from build123d import *

# Parameters (mm, degrees)
SKETCH1_R           = 2.921
BOSS_EXTRUDE1_DEPTH = 2.54
SKETCH3_R           = 0.762
CUT_EXTRUDE1_DEPTH  = 0.254
FILLET1_R           = 1.27
SCALE1_SCALE        = 2.43
SCALE3_SCALE        = 1.15


with BuildPart() as part:
    # Sketch1 → Boss-Extrude1 (new body)
    with BuildSketch(Plane.XY):
        with BuildLine():
            Line((0, 0), (5.08, 0))
            ThreePointArc((5.08, 0), (5.715, 6.285851973), (3.835659211, 0.254))
            Line((3.835659211, 0.254), (0, 0.254))
            Line((0, 0.254), (0, 0))
        make_face()
        with Locations((5.08, 3.175)):
            Circle(SKETCH1_R, mode=Mode.SUBTRACT)
    extrude(amount=BOSS_EXTRUDE1_DEPTH)

    # Sketch3 → Cut-Extrude1 (cut)
    with BuildSketch(Plane(origin=(0, 0.254, 0), x_dir=(1, 0, 0), z_dir=(0, 1, 0))):
        with Locations(Location((1.4605, -1.27, 0), (0, 0, 180))):
            Circle(SKETCH3_R)
    extrude(amount=-CUT_EXTRUDE1_DEPTH, mode=Mode.SUBTRACT)

    # Fillet1
    fillet1_edges = [part.edges().sort_by_distance(p)[0] for p in [
        (0, 0.127, 2.54),
        (0, 0.127, 0),
    ]]
    fillet(fillet1_edges, radius=FILLET1_R - 0.0001)  # a hair under: the kernel refuses the full size


with BuildPart() as part_1:
    # Scale1: scaled about (4.695948506, 2.731518553, 1.27)
    add(part.part.scale(SCALE1_SCALE).moved(Location((-6.715206364, -3.906071531, -1.8161))))


with BuildPart() as part_2:
    # Scale3: scaled about (4.695948505, 2.731518554, 1.27)
    add(part_1.part.scale(SCALE3_SCALE).moved(Location((-0.704392276, -0.409727783, -0.1905))))


solid = part_2.part
Could you check a few things on this model? Use its own coordinates, in mm. A direction names the side the tool comes from. Give positions to 0.01 mm unless a question says otherwise; leave off trailing zeros. Loops run counter-clockwise (first coordinate to the right, second up) from the corner with the lowest first, then second, coordinate; pieces in that order, holes last. Notation, with made-up numbers: (-10, 29.5) -> (7, 29.5) arc R21 ccw to (7, 67.5) -> close; hole circle Ø7 at (42.5, 82.5). An arc over 180 degrees is marked (long way). Return JSON: item names as keys, results as strings.
Item 1: We'd pull the mould along X, two halves only. Please class faces 4 (the cylindrical face through (-7.415, -4.552, -1.212)), 5 (the flat face through (0, -4.902, 1)), 6 (the cylindrical face through (-0.708, -0.996, 1.22)): +X half, -X half, draft (parallel to the pull), parting line (faces both ways), or undercut.
Geometry results:
{"face 4": "-X half", "face 5": "draft", "face 6": "undercut"}
Item 2: Which directions (+Z, -Z, +X, -X, +Y, -Y) give clear straight access to the entire face, cutting with the end or side of a thin tool? Please do faces 1 (the flat face through (-2, -4.192, 1)), 2 (the cylindrical face through (-6.31, -4.54, 0.45)), 3 (the flat face through (3, -4, 4.819)).
Geometry results:
{"face 1": "+Z, -Z, -X", "face 2": "-Y", "face 3": "+Z, +X, -X, +Y, -Y"}
Item 3: I'm going to push flat-ended pins straight in: pin 1 (8 mm diameter, centred on x = -4, y = 2.5, fed in from -Z); pin 2 (3 mm diameter, centred on y = 8, z = -1.5, fed in from -X); pin 3 (1 mm diameter, centred on y = 1, z = 4, fed in from +X); pin 4 (10 mm diameter, centred on x = 5.5, y = 5, fed in from +Z). Where does each tip first touch, or does it pass through?
Geometry results:
{"pin 1": "stops at z = -2.28", "pin 2": "stops at x = -2.74", "pin 3": "stops at x = 14.29", "pin 4": "passes through"}
Item 4: If we section it at C-C on x = 4.5: List the corners of the cut face in (y, z) for me.
Geometry results:
{"outline": "(-4.9, -2.28) -> (-4.09, -2.28) -> (-4.09, 4.82) -> (-4.9, 4.82) -> close; (12.03, -2.28) -> (12.75, -2.28) -> (12.75, 4.82) -> (12.03, 4.82) -> close"}
Item 5: If we section it at A-A on z = 2: List the corners of the cut face in (x, y) for me.
Geometry results:
{"outline": "(-8.35, -4.9) -> (-6.35, -4.9) -> (-6.35, -4.19) -> (-8.35, -4.19) -> close; (-2.35, -4.9) -> (5.77, -4.9) arc R8.87 ccw (long way) to (2.29, -4.19) -> (-2.35, -4.19) -> close; hole circle Ø16.33 at (5.77, 3.97)"}
Item 6: I need wall thicknesses on L1, parallel to Y at x = 5.5, z = 3.25; L2, parallel to Y at x = 0.25, z = 3.5; L3, parallel to Y at x = -1.5, z = 0.5. Which ranges of each line are inside material? Lowest first, please. Write a range as from..to.
Geometry results:
{"L1": "y = -4.9..-4.19, 12.13..12.84", "L2": "y = -4.9..-4.19, -2.98..-2.04, 9.98..10.92", "L3": "y = -4.9..-4.19, -1.12..0.26, 7.68..9.06"}
Item 7: If we section it at D-D on z = 0.5: List the corners of the cut face in (x, y) for me, plus the area to 3 significant figures.
Geometry results:
{"outline": "(-8.34, -4.9) -> (-6.33, -4.9) -> (-6.33, -4.19) -> (-8.34, -4.19) -> close; (-2.36, -4.9) -> (5.77, -4.9) arc R8.87 ccw (long way) to (2.29, -4.19) -> (-2.36, -4.19) -> close; hole circle Ø16.33 at (5.77, 3.97)", "area": "43.5 mm²"}
Item 8: If we section it at B-B on y = 5: List the corners of the cut face in (x, z) for me.
Geometry results:
{"outline": "(-3.04, -2.28) -> (-2.33, -2.28) -> (-2.33, 4.82) -> (-3.04, 4.82) -> close; (13.87, -2.28) -> (14.58, -2.28) -> (14.58, 4.82) -> (13.87, 4.82) -> close"}
